Design review of the part built by this model. Coordinates are the model's own, in mm. Coordinates: 2 decimals unless noted, no trailing zeros. Write each loop counter-clockwise with the first axis right and the second up, starting at its lowest first coordinate (ties: lowest second). Pieces come first, ordered by that corner, then holes. Notation, with made-up numbers: (31.25, 20.5) -> (89.25, 20.5) arc R26 ccw to (89.25, 41.5) -> close; hole circle Ø9 at (55.25, -6.75). An arc over 180 degrees is marked (long way). One line per question, with ' | ' between items. Start each with the question number.
Q1. Draft analysis for pull direction Y (two halves, no side actions). For faces 1 (the cylindrical face through (136.993, -139.273, 5.07)), 2 (the cylindrical face through (-137.148, 139.118, 5.07)), 3 (the cylindrical face through (-123.88, -120.52, 5.07)), state which applies: pulls with the +Y half, pulls with the -Y half, needs draft (parallel to the pull), parting line crosses it, or undercut.
Q2. Add section A-A on x = -120. State the section outline as (y, z) points (3 decimals).
Q3. Wall thickness on probe 1 along Y at (x, z) = (-120, 8.25) (3 decimals): over which ranges is the line inside the solid? List them lowest first.
Q4. For P1, Ø5, axis at x = -120, y = 122.125, coming from the -Z side, flat-tipped, find the tip position at first contact; note if it passes through.
from build123d import *

# Parameters (mm, degrees)
SKETCH_1_W              = 280
SKETCH_1_H              = 284.25
EXTRUDE_1_DEPTH         = 10
FILLET_1_R              = 10
HOLE_WIZARD_8_4_8_4_1_D = 8.4


with BuildPart() as part:
    # 草图1 → 凸台-拉伸1 (new body)
    with BuildSketch(Plane.XY):
        Rectangle(SKETCH_1_W, SKETCH_1_H)
    extrude(amount=EXTRUDE_1_DEPTH)

    # 圆角1
    fillet_1_edges = [part.edges().sort_by_distance(p)[0] for p in [
        (140, -142.125, 5),
        (-140, -142.125, 5),
        (-140, 142.125, 5),
        (140, 142.125, 5),
    ]]
    fillet(fillet_1_edges, radius=FILLET_1_R)

    # Ø8.4 (8.4) 直径孔1 (through all)
    with Locations(Plane(origin=(0, 0, 0), x_dir=(1, 0, 0), z_dir=(0, 0, -1))):
        with Locations((-120, -122.125), (120, -122.125), (120, 122.125), (-120, 122.125)):
            Hole(HOLE_WIZARD_8_4_8_4_1_D / 2)


solid = part.part
Output values:
1) face 1: pulls with the -Y half | face 2: pulls with the +Y half | face 3: undercut
2) outline: (-142.125, 0) -> (-126.325, 0) -> (-126.325, 10) -> (-142.125, 10) -> close; (-117.925, 0) -> (117.925, 0) -> (117.925, 10) -> (-117.925, 10) -> close; (126.325, 0) -> (142.125, 0) -> (142.125, 10) -> (126.325, 10) -> close
3) probe 1: y = -142.125 to -126.325, -117.925 to 117.925, 126.325 to 142.125
4) P1: passes through
